from build123d import *

# Parameters (mm, degrees)
PAD_DEPTH       = 3
SKETCH001_R     = 2.125
POCKET_DEPTH    = 2.15
CHAMFER_SIZE    = 0.2
CHAMFER001_SIZE = 0.2
SKETCH002_W     = 1.5
SKETCH002_H     = 7
PAD001_DEPTH    = 8
FILLET_R        = 0.5
FILLET001_R     = 1


with BuildPart() as part:
    # Sketch → Pad (new body)
    with BuildSketch(Plane.XY):
        Polygon((4.618802, 0), (2.309401, 4), (-2.309401, 4), (-4.618802, 0), (-2.309401, -4), (2.309401, -4), align=None)
    extrude(amount=PAD_DEPTH)

    # Sketch001 → Pocket (cut)
    with BuildSketch(Plane.XY):
        Circle(SKETCH001_R)
    extrude(amount=POCKET_DEPTH, mode=Mode.SUBTRACT)

    # Chamfer
    chamfer_edges = [part.edges().sort_by_distance(p)[0] for p in [
        (3.464102, 2, 3),
        (0, 4, 3),
        (-3.464102, 2, 3),
        (-3.464102, -2, 3),
        (0, -4, 3),
        (3.464102, -2, 3),
    ]]
    chamfer(chamfer_edges, length=CHAMFER_SIZE)

    # Chamfer001
    chamfer001_edges = [part.edges().sort_by_distance(p)[0] for p in [
        (3.464102, 2, 0),
        (3.464102, -2, 0),
        (0, 4, 0),
        (0, -4, 0),
        (-3.464102, 2, 0),
        (-3.464102, -2, 0),
        (-2.125, 0, 0),
    ]]
    chamfer(chamfer001_edges, length=CHAMFER001_SIZE)

    # Sketch002 (on Face11 of Chamfer001) → Pad001 (join)
    with BuildSketch(Plane.XY.offset(3)):
        with Locations((-0.75, 0)):
            Rectangle(SKETCH002_W, SKETCH002_H)
    extrude(amount=PAD001_DEPTH)

    # Fillet
    fillet_edges = [part.edges().sort_by_distance(p)[0] for p in [
        (-1.5, 0, 3),
    ]]
    fillet(fillet_edges, radius=FILLET_R)

    # Fillet001
    fillet001_edges = [part.edges().sort_by_distance(p)[0] for p in [
        (-0.75, -3.5, 11),
        (-0.75, 3.5, 11),
    ]]
    fillet(fillet001_edges, radius=FILLET001_R)


solid = part.part
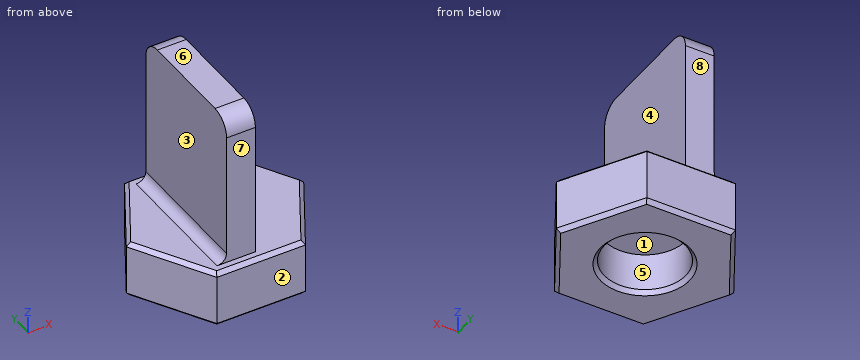
Part model, mm, in its own coordinate system. Face numbers are marked on the shaded views. A direction names the side the tool comes from. Coordinates: 2 decimals unless noted, no trailing zeros. Loops run counter-clockwise (first coordinate to the right, second up) from the corner with the lowest first, then second, coordinate; pieces in that order, holes last. Notation, with made-up numbers: (-13, 2.5) - (35, 2.5) arc R13 cw to (35, 17.5) - close; hole circle Ø11 at (63, 34). An arc over 180 degrees is marked (long way). Write each question's results on one line, items separated by ' | '. Start each with the question number.
Q1. Two-plate mould, pull along X, no slides. Class the marked faces 1, 2 and 3: +X half, -X half, draft (parallel to the pull), parting line (faces both ways), or undercut.
Q2. Probe line 1 along Y through (x, z) = (0, 1.55) (3 decimals); line 2 along X through (y, z) = (-1.5, 7.5); line 3 along Z through (x, y) = (3, -1). List the from-to ranges inside material, lowest first.
Q3. Slice it at A-A on z = 1.25. Give the cut face in (x, y) (3 decimals), and give its area (3 significant figures).
Q4. Slice it at C-C on x = 4. Give the cut face in (y, z).
Q5. Slice it at D-D on z = 7.25. Give the cut face in (x, y).
Q6. Slice it at B-B on y = 3. Give the cut face in (x, z).
Q7. Which spindle directions (+Z, -Z, +X, -X, +Y, -Y) get a long thin tool onto all of the face, cutting with end or side? Do the marked faces 4, 5, 6, 7 and 8. Say none if no direction does.
Q8. Drop flat-ended pins along their axis: pin 1 Ø2 at (x, y) = (-0.5, 0.5) entering from -Z; pin 2 Ø3.5 at (y, z) = (1, 7.5) entering from -X; pin 3 Ø2 at (y, z) = (1, 8.5) entering from +X. Give the stop position or say it passes through.
Answer:
1) face 1: undercut | face 2: draft | face 3: -X half
2) line 1: y = -4 to -2.125, 2.125 to 4 | line 2: x = -1.5 to 0 | line 3: z = 0 to 3
3) outline: (-4.619, 0) - (-2.309, -4) - (2.309, -4) - (4.619, 0) - (2.309, 4) - (-2.309, 4) - close; hole circle Ø4.25 at (0, 0) | area: 41.2 mm2
4) outline: (-1.07, 0.2) - (-0.67, 0) - (0.67, 0) - (1.07, 0.2) - (1.07, 2.8) - (0.67, 3) - (-0.67, 3) - (-1.07, 2.8) - close
5) outline: (-1.5, -3.5) - (0, -3.5) - (0, 3.5) - (-1.5, 3.5) - close
6) outline: (-2.89, 0.2) - (-2.66, 0) - (2.66, 0) - (2.89, 0.2) - (2.89, 2.8) - (2.66, 3) - (0, 3) - (0, 10.87) - (-1.5, 10.87) - (-1.5, 3.5) arc R0.5 cw to (-2, 3) - (-2.66, 3) - (-2.89, 2.8) - close
7) face 4: +Z, +X, +Y, -Y | face 5: -Z | face 6: +Z, +X, -X, +Y, -Y | face 7: +Z, +X, -X, -Y | face 8: +Z, +X, -X, +Y
8) pin 1: stops at z = 2.15 | pin 2: stops at x = -1.5 | pin 3: stops at x = 0
